Can you work these out from the model? Positions are in its coordinate system, mm. Face numbers are marked on the shaded views. A direction names the side the tool comes from. Coordinates: 2 decimals unless noted, no trailing zeros. Order: outer loops, then holes, each group sorted by start corner. A loop starts at its lowest first (then second) coordinate and runs counter-clockwise, first axis right, second up.
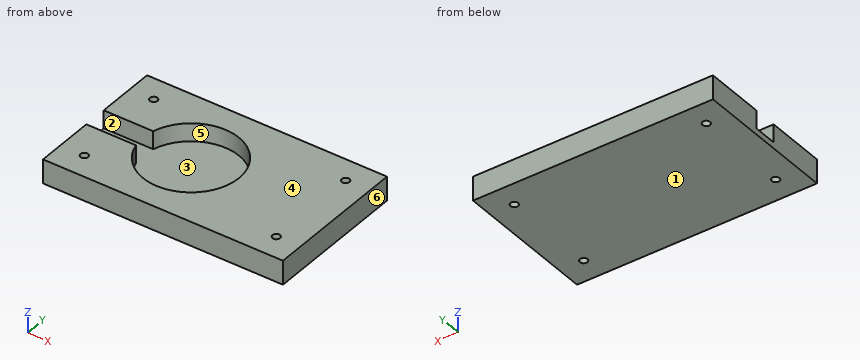
```python
from build123d import *

# Parameters (mm, degrees)
SKETCH_W                = 254
SKETCH_H                = 152.4
PAD_DEPTH               = 25.4
SKETCH001_R             = 4
POCKET_DEPTH            = 619.999755
SKETCH001_MIRRORED_2_R  = 4
POCKET_MIRRORED_2_DEPTH = 619.999755
POCKET001_DEPTH         = 19.05


with BuildPart() as part:
    # Sketch → Pad (new body)
    with BuildSketch(Plane.XY):
        Rectangle(SKETCH_W, SKETCH_H)
    extrude(amount=PAD_DEPTH)

    # Sketch001 (on Face6 of Pad) → Pocket (cut, through all)
    with BuildSketch(Plane.XY.offset(25.4)):
        with Locations((-101.6, 50.8)):
            Circle(SKETCH001_R)
    pocket = extrude(amount=-POCKET_DEPTH, mode=Mode.SUBTRACT)

    # Sketch001 Mirrored 2 → Pocket Mirrored 2 (cut, through all)
    with BuildSketch(Plane(origin=(0, 0, 25.4), x_dir=(-1, 0, 0), z_dir=(0, 0, -1))):
        with Locations((-101.6, 50.8)):
            Circle(SKETCH001_MIRRORED_2_R)
    pocket_mirrored_2 = extrude(amount=POCKET_MIRRORED_2_DEPTH, mode=Mode.SUBTRACT)

    # Mirrored001: Pocket, Pocket Mirrored 2 across XZ
    add(pocket.mirror(Plane.XZ), mode=Mode.SUBTRACT)
    add(pocket_mirrored_2.mirror(Plane.XZ), mode=Mode.SUBTRACT)

    # Sketch002 (on Face5 of MultiTransform) → Pocket001 (cut)
    with BuildSketch(Plane.XY.offset(25.4)):
        with BuildLine():
            Line((-127, -12.7), (-74.586888, -12.7))
            ThreePointArc((-74.586888, -12.7), (25.4, 0), (-74.586888, 12.7))
            Line((-74.586888, 12.7), (-127, 12.7))
            Line((-127, 12.7), (-127, -12.7))
        make_face()
    extrude(amount=-POCKET001_DEPTH, mode=Mode.SUBTRACT)


solid = part.part
```
1. Thinking about a two-plate mould opening in X: for the marked faces 3, 4, 5 and 6, which applies, pulls with the +X half, pulls with the -X half, needs draft (parallel to the pull), parting line crosses it, or undercut?
Completed:
face 3: undercut
face 4: needs draft
face 5: undercut
face 6: pulls with the +X half
2. I'm going to push flat-ended pins straight in: pin 1 (6.5 mm diameter, centred on x = 101.6, y = -50.8, fed in from -Z); pin 2 (6 mm diameter, centred on y = -7.5, z = 14.5, fed in from -X). Where does each tip first touch, or does it pass through?
Completed:
pin 1: passes through
pin 2: stops at x = 24.3
3. Imagine slicing it at A-A on z = 11.5. Please give me the cut outline in (x, y), then the cut area to 3 significant figures.
Completed:
outline: (-127, -76.2) - (127, -76.2) - (127, 76.2) - (-127, 76.2) - (-127, 12.7) - (-74.59, 12.7) arc R50.8 cw (long way) to (-74.59, -12.7) - (-127, -12.7) - close; hole circle Ø8 at (-101.6, -50.8); hole circle Ø8 at (-101.6, 50.8); hole circle Ø8 at (101.6, -50.8); hole circle Ø8 at (101.6, 50.8)
area: 29,100 mm2
4. Imagine slicing it at D-D on y = 0. Please give me the cut outline in (x, z).
Completed:
outline: (-127, 0) - (127, 0) - (127, 25.4) - (25.4, 25.4) - (25.4, 6.35) - (-127, 6.35) - close
5. Imagine slicing it at C-C on x = -25.4. Please give me the cut outline in (y, z), then the cut area to 3 significant figures.
Completed:
outline: (-76.2, 0) - (76.2, 0) - (76.2, 25.4) - (50.8, 25.4) - (50.8, 6.35) - (-50.8, 6.35) - (-50.8, 25.4) - (-76.2, 25.4) - close
area: 1,940 mm2
6. Imagine slicing it at B-B on x = -101.6. Please give me the cut outline in (y, z), then the cut area to 3 significant figures.
Completed:
outline: (-76.2, 0) - (-54.8, 0) - (-54.8, 25.4) - (-76.2, 25.4) - close; (-46.8, 0) - (46.8, 0) - (46.8, 25.4) - (12.7, 25.4) - (12.7, 6.35) - (-12.7, 6.35) - (-12.7, 25.4) - (-46.8, 25.4) - close; (54.8, 0) - (76.2, 0) - (76.2, 25.4) - (54.8, 25.4) - close
area: 2,980 mm2
7. On a 3-axis mill with a long thin cutter (end or side, diameter ignored), from which of +Z, -Z, +X, -X, +Y, -Y can I reach the whole of each face in a straight line? I mean the marked faces 1 and 2. Say none if no direction works.
Completed:
face 1: -Z, +X, -X, +Y, -Y
face 2: +Z, -X
8. Please list where these lines run through material, in increasing order: probe 1 along Y at (x, z) = (101.6, 12); probe 2 along Z at (x, y) = (-4.5, 27.5); probe 3 along X at (y, z) = (0, 17.75).
Completed:
probe 1: y = -76.2 to -54.8, -46.8 to 46.8, 54.8 to 76.2
probe 2: z = 0 to 6.35
probe 3: x = 25.4 to 127
